from build123d import *

# Parameters (mm, degrees)
CROQUIS1_R              = 10
CROQUIS1_W              = 3
CROQUIS1_H              = 3
SALIENTE_EXTRUIR2_DEPTH = 3


with BuildPart() as part:
    # Croquis1 → Saliente-Extruir2 (new body)
    with BuildSketch(Plane(origin=(0, 0, 0), x_dir=(1, 0, 0), z_dir=(0, 1, 0))):
        Polygon((-72, -72), (-65, -72), (-65, -75), (-55, -75), (-55, -72), (-45, -72), (-45, -75), (-35, -75), (-35, -72), (-25, -72), (-25, -75), (-15, -75), (-15, -72), (-5, -72), (-5, -75), (5, -75), (5, -72), (15, -72), (15, -75), (25, -75), (25, -72), (35, -72), (35, -75), (45, -75), (45, -72), (55, -72), (55, -75), (65, -75), (65, -72), (72, -72), (72, -65), (75, -65), (75, -55), (72, -55), (72, -45), (75, -45), (75, -35), (72, -35), (72, -25), (75, -25), (75, -15), (72, -15), (72, -5), (75, -5), (75, 5), (72, 5), (72, 15), (75, 15), (75, 25), (72, 25), (72, 35), (75, 35), (75, 45), (72, 45), (72, 55), (75, 55), (75, 65), (72, 65), (72, 72), (65, 72), (65, 75), (55, 75), (55, 72), (45, 72), (45, 75), (35, 75), (35, 72), (25, 72), (25, 75), (15, 75), (15, 72), (5, 72), (5, 75), (-5, 75), (-5, 72), (-15, 72), (-15, 75), (-25, 75), (-25, 72), (-35, 72), (-35, 75), (-45, 75), (-45, 72), (-55, 72), (-55, 75), (-65, 75), (-65, 72), (-72, 72), (-72, 65), (-75, 65), (-75, 55), (-72, 55), (-72, 45), (-75, 45), (-75, 35), (-72, 35), (-72, 25), (-75, 25), (-75, 15), (-72, 15), (-72, 5), (-75, 5), (-75, -5), (-72, -5), (-72, -15), (-75, -15), (-75, -25), (-72, -25), (-72, -35), (-75, -35), (-75, -45), (-72, -45), (-72, -55), (-75, -55), (-75, -65), (-72, -65), align=None)
        with Locations(Location((0, 0, 0), (0, 0, 270))):
            Circle(CROQUIS1_R, mode=Mode.SUBTRACT)
        with Locations((18.5, 23.5)):
            Rectangle(CROQUIS1_W, CROQUIS1_H, mode=Mode.SUBTRACT)
        with Locations((-18.5, 23.5)):
            Rectangle(CROQUIS1_W, CROQUIS1_H, mode=Mode.SUBTRACT)
        with Locations((-23.5, 18.5)):
            Rectangle(CROQUIS1_W, CROQUIS1_H, mode=Mode.SUBTRACT)
        with Locations((-23.5, -18.5)):
            Rectangle(CROQUIS1_W, CROQUIS1_H, mode=Mode.SUBTRACT)
        with Locations((23.5, -18.5)):
            Rectangle(CROQUIS1_W, CROQUIS1_H, mode=Mode.SUBTRACT)
        with Locations((23.5, 18.5)):
            Rectangle(CROQUIS1_W, CROQUIS1_H, mode=Mode.SUBTRACT)
        with Locations((18.5, -23.5)):
            Rectangle(CROQUIS1_W, CROQUIS1_H, mode=Mode.SUBTRACT)
        with Locations((-18.5, -23.5)):
            Rectangle(CROQUIS1_W, CROQUIS1_H, mode=Mode.SUBTRACT)
    extrude(amount=SALIENTE_EXTRUIR2_DEPTH)


solid = part.part
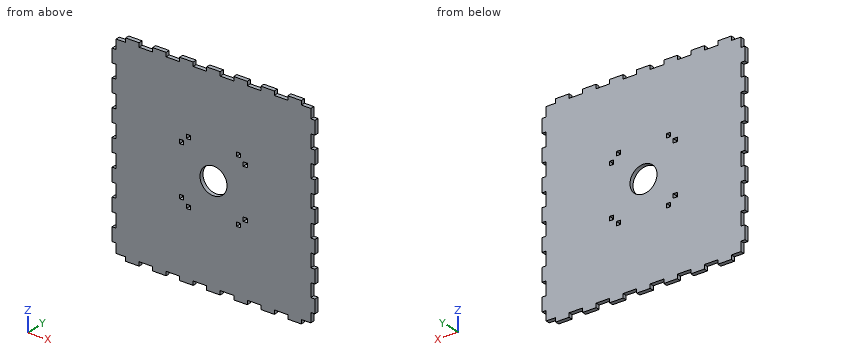
Work out the finished part from the listing and answer in its coordinate system (mm). Round coordinates to 2 decimals unless told otherwise and drop trailing zeros. Write each loop counter-clockwise with the first axis right and the second up, starting at its lowest first coordinate (ties: lowest second). Pieces come first, ordered by that corner, then holes.
1) A cutting plane is placed at D-D (x = 29). Give the vertices of the cut face in (y, z).
2) A cutting plane is placed at C-C (y = 0.5). Give the number of separate pieces and of enclosed holes in the cut face, plus the area to 3 significant figures.
3) A cutting plane is placed at A-A (z = 0). Give the vertices of the cut face in (x, y), plus the area to 3 significant figures.
4) A cutting plane is placed at B-B (x = 0). Give the vertices of the cut face in (y, z).
5) Given pin 1 Ø1.5 at (x, y) = (74, 1.5) entering from +Z; pin 2 Ø1 at (x, y) = (-29, 1.5) entering from +Z; pin 3 Ø0.9 at (x, y) = (74, 1) entering from -Z, each flat-ended and moving along its own axis, determine where each tip first touches the part or whether it passes through.
6) Straight lines are drawn through the part: line 1 (Z direction, x = 17.5, y = 0.4); line 2 (X direction, y = 1.75, z = 0); line 3 (X direction, y = 2.2, z = 11). For each, find the intervals that lie inside material, in ascending order.
Completed:
1. outline: (0, -72) - (3, -72) - (3, 72) - (0, 72) - close
2. separate pieces: 1
2. enclosed holes: 9
2. area: 21,200 mm2
3. outline: (-75, 0) - (-10, 0) - (-10, 3) - (-75, 3) - close; (10, 0) - (75, 0) - (75, 3) - (10, 3) - close
3. area: 390 mm2
4. outline: (0, -75) - (3, -75) - (3, -10) - (0, -10) - close; (0, 10) - (3, 10) - (3, 75) - (0, 75) - close
5. pin 1: stops at z = 65
5. pin 2: stops at z = 72
5. pin 3: stops at z = -65
6. line 1: z = -75 to -25, -22 to 22, 25 to 75
6. line 2: x = -75 to -10, 10 to 75
6. line 3: x = -72 to 72
